from build123d import *

# Parameters (mm, degrees)
F1_DEPTH       = 8
F3_D           = 3.3
F3_CSINK_D     = 6.72
F3_CSINK_ANGLE = 90
F4_DEPTH       = 12
F5_DEPTH       = 4
F6_R           = 3


with BuildPart() as f1:
    # F0 (on Top) → F1 (new body)
    with BuildSketch(Plane.XY):
        Polygon((44.2503372943, 75.0596572278), (6.9678689315, 21.814774349), (16.7340656416, 21.814774349), (48.4148736987, 67.0596572278), (54.2503372943, 67.0596572278), (54.2503372943, 75.0596572278), align=None)
    extrude(amount=F1_DEPTH)

    # F3 (through all)
    with Locations(Plane(origin=(0, 75.0596572278, 0), x_dir=(-1, 0, 0), z_dir=(0, 1, 0))):
        with Locations((-49.2503372943, 4)):
            CounterSinkHole(F3_D / 2, F3_CSINK_D / 2, counter_sink_angle=F3_CSINK_ANGLE)

    # F0 (on Top) → F4 (join)
    with BuildSketch(Plane.XY):
        Polygon((16.7340656416, 21.814774349), (6.9678689315, 21.814774349), (6.9678689315, 11.814774349), (16.9678689315, 11.814774349), (16.9678689315, 21.814774349), align=None)
        Polygon((6.9678689315, 11.814774349), (6.9678689315, 21.814774349), (-33.0321310685, 21.814774349), (-33.0321310685, 1.814774349), (-25.0321310685, 1.814774349), (-25.0321310685, 16.814774349), (-6.0321310685, 16.814774349), (-6.0321310685, 1.814774349), (16.9678689315, 1.814774349), (16.9678689315, 11.814774349), align=None)
    extrude(amount=F4_DEPTH)

    # F0 (on Top) → F5 (join)
    with BuildSketch(Plane.XY):
        Polygon((6.9678689315, 11.814774349), (6.9678689315, 21.814774349), (-33.0321310685, 21.814774349), (-33.0321310685, 1.814774349), (-25.0321310685, 1.814774349), (-25.0321310685, 16.814774349), (-6.0321310685, 16.814774349), (-6.0321310685, 1.814774349), (16.9678689315, 1.814774349), (16.9678689315, 11.814774349), align=None)
        Polygon((16.7340656416, 21.814774349), (6.9678689315, 21.814774349), (6.9678689315, 11.814774349), (16.9678689315, 11.814774349), (16.9678689315, 21.814774349), align=None)
    extrude(amount=-F5_DEPTH)

    # F6
    f6_edges = [f1.edges().sort_by_distance(p)[0] for p in [
        (54.250337, 71.059657, 0),
        (54.250337, 71.059657, 8),
    ]]
    fillet(f6_edges, radius=F6_R)


solid = f1.part
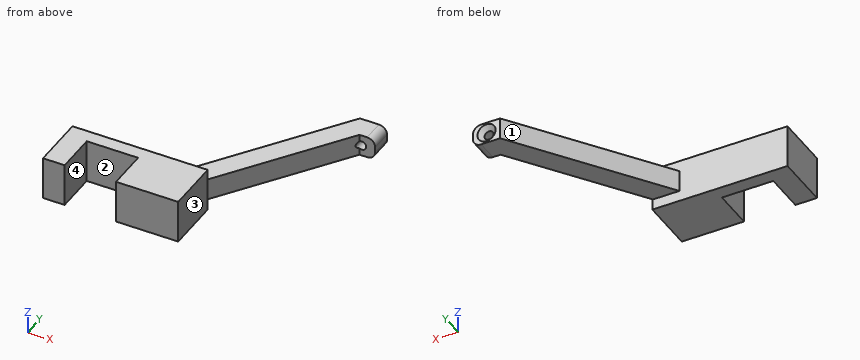
Read the model definition and answer for the solid it produces. Units are mm, in the model's axes. Face numbers are marked on the shaded views. Round coordinates to 2 decimals unless told otherwise and drop trailing zeros. Order: outer loops, then holes, each group sorted by start corner. A loop starts at its lowest first (then second) coordinate and runs counter-clockwise, first axis right, second up.
1) The mould has two halves that part along X. Classify the marked faces 1, 2, 3 and 4: released by +X, released by -X, zero draft, split by the parting line, or undercut.
2) The part is cut by section A-A on z = 4. Write down the section's boundary in (x, y), plus the area to 3 significant figures.
3) The part is cut by section D-D on y = 44. Write down the section's boundary in (x, z).
4) Straight lines are drawn through the part: L1, parallel to X at y = 9, z = 2.25; L2, parallel to X at y = 19.5, z = 10; L3, parallel to X at y = 71.5, z = 4. For each, find the intervals that lie inside material, in ascending order.
5) The part is cut by section C-C on z = -2.25. Write down the section's boundary in (x, y), plus the area to 3 significant figures.
6) Flat-ended cylindrical pins translate along their axes: pin 1 (13.5 mm diameter, centred on x = 38, y = 58.5, fed in from +Z); pin 2 (5 mm diameter, centred on y = 34.5, z = 4.5, fed in from -X); pin 3 (7.5 mm diameter, centred on y = 6, z = 4, fed in from +X). Find the tip coordinate at first contact, or state that the pin passes through.
7) The part is cut by section B-B on x = 13. Write down the section's boundary in (y, z).
Resolved:
1. face 1: released by -X
1. face 2: undercut
1. face 3: released by +X
1. face 4: undercut
2. outline: (-33.03, 1.81) - (-25.03, 1.81) - (-25.03, 16.81) - (-6.03, 16.81) - (-6.03, 1.81) - (16.97, 1.81) - (16.97, 21.81) - (16.73, 21.81) - (47.6, 65.9) - (47.6, 73.35) - (45.89, 75.06) - (44.25, 75.06) - (6.97, 21.81) - (-33.03, 21.81) - close; (50.9, 67.06) - (54.25, 67.06) - (54.25, 75.06) - (52.61, 75.06) - (50.9, 73.35) - close
2. area: 1,230 mm2
3. outline: (22.5, 0) - (32.27, 0) - (32.27, 8) - (22.5, 8) - close
4. L1: x = -33.03 to -25.03, -6.03 to 16.97
4. L2: x = -33.03 to 16.97
4. L3: x = 41.76 to 47.6, 50.9 to 54.25
5. outline: (-33.03, 1.81) - (-25.03, 1.81) - (-25.03, 16.81) - (-6.03, 16.81) - (-6.03, 1.81) - (16.97, 1.81) - (16.97, 21.81) - (-33.03, 21.81) - close
5. area: 715 mm2
6. pin 1: stops at z = 8
6. pin 2: stops at x = 14.1
6. pin 3: stops at x = 16.97
7. outline: (1.81, -4) - (21.81, -4) - (21.81, 0) - (30.43, 0) - (30.43, 8) - (21.81, 8) - (21.81, 12) - (1.81, 12) - close
